from build123d import *

# Parameters (mm, degrees)
SKETCH1_W            = 103
SKETCH1_H            = 62.04
BOSS_EXTRUDE1_DEPTH  = 2
SKETCH2_W            = 103
SKETCH2_H            = 2
BOSS_EXTRUDE2_DEPTH  = 3
SKETCH5_W            = 8
SKETCH5_H            = 2.5
BOSS_EXTRUDE4_DEPTH  = 10
BOSS_EXTRUDE5_DEPTH  = 10
SKETCH7_R            = 1
CUT_EXTRUDE1_DEPTH   = 3
FILLET2_R            = 2
SKETCH8_W            = 103
SKETCH8_H            = 2.5
BOSS_EXTRUDE6_DEPTH  = 3
SKETCH9_W            = 8
SKETCH9_H            = 2.5
BOSS_EXTRUDE7_DEPTH  = 2
SKETCH11_R           = 1
CUT_EXTRUDE3_DEPTH   = 22
FILLET4_R            = 1
SKETCH12_W           = 12
SKETCH12_H           = 2.5
BOSS_EXTRUDE8_DEPTH  = 2
FILLET5_R            = 1
SKETCH13_R           = 0.95132711
CUT_EXTRUDE4_DEPTH   = 12
FILLET6_R            = 1
SKETCH14_W           = 103
SKETCH14_H           = 2.5
BOSS_EXTRUDE9_DEPTH  = 3
SKETCH15_W           = 8
SKETCH15_H           = 2.5
BOSS_EXTRUDE10_DEPTH = 5
SKETCH16_R           = 1
CUT_EXTRUDE5_DEPTH   = 15
FILLET7_R            = 1
CUT_EXTRUDE6_DEPTH   = 5


with BuildPart() as part:
    # Sketch1 → Boss-Extrude1 (new body)
    with BuildSketch(Plane(origin=(0, 0, 0), x_dir=(1, 0, 0), z_dir=(0, 1, 0))):
        Rectangle(SKETCH1_W, SKETCH1_H)
    extrude(amount=BOSS_EXTRUDE1_DEPTH)

    # Sketch2 → Boss-Extrude2 (add)
    with BuildSketch(Plane(origin=(0, 0, -31.02), x_dir=(-1, 0, 0), z_dir=(0, 0, -1))):
        with Locations((0, 1)):
            Rectangle(SKETCH2_W, SKETCH2_H)
    extrude(amount=BOSS_EXTRUDE2_DEPTH)

    # Sketch5 → Boss-Extrude4 (add)
    with BuildSketch(Plane(origin=(0, 2, 0), x_dir=(1, 0, 0), z_dir=(0, 1, 0))):
        with Locations((47.5, 29.77)):
            Rectangle(SKETCH5_W, SKETCH5_H)
    boss_extrude4 = extrude(amount=BOSS_EXTRUDE4_DEPTH)

    # Sketch6 → Boss-Extrude5 (add)
    with BuildSketch(Plane(origin=(0, 2, 0), x_dir=(1, 0, 0), z_dir=(0, 1, 0))):
        Polygon((43.5, 28.52), (0, 28.52), (0, 30.925842428), (43.5, 31.02), align=None)
    boss_extrude5 = extrude(amount=BOSS_EXTRUDE5_DEPTH)

    # Sketch7 → Cut-Extrude1 (cut)
    with BuildSketch(Plane.XY.offset(-28.52)):
        with Locations((47.5, 6)):
            Circle(SKETCH7_R)
    cut_extrude1 = extrude(amount=-CUT_EXTRUDE1_DEPTH, mode=Mode.SUBTRACT)

    # Mirror1: Boss-Extrude4, Boss-Extrude5, Cut-Extrude1 across plane
    add(boss_extrude4.mirror(Plane(origin=(0, 0, 0), x_dir=(0, 0, 1), z_dir=(1, 0, 0))))
    add(boss_extrude5.mirror(Plane(origin=(0, 0, 0), x_dir=(0, 0, 1), z_dir=(1, 0, 0))))
    add(cut_extrude1.mirror(Plane(origin=(0, 0, 0), x_dir=(0, 0, 1), z_dir=(1, 0, 0))), mode=Mode.SUBTRACT)

    # Fillet2
    fillet2_edges = [part.edges().sort_by_distance(p)[0] for p in [
        (0, 2, -28.52),
    ]]
    fillet(fillet2_edges, radius=FILLET2_R)

    # Sketch8 → Boss-Extrude6 (add)
    with BuildSketch(Plane(origin=(0, 2, 0), x_dir=(1, 0, 0), z_dir=(0, 1, 0))):
        with Locations((0, -3.73)):
            Rectangle(SKETCH8_W, SKETCH8_H)
    extrude(amount=BOSS_EXTRUDE6_DEPTH)

    # Sketch9 → Boss-Extrude7 (add)
    with BuildSketch(Plane(origin=(0, 5, 0), x_dir=(1, 0, 0), z_dir=(0, 1, 0))):
        with Locations((47.5, -3.73)):
            Rectangle(SKETCH9_W, SKETCH9_H)
    extrude(amount=BOSS_EXTRUDE7_DEPTH)

    # Sketch11 → Cut-Extrude3 (cut)
    with BuildSketch(Plane.XY.offset(4.98)):
        with Locations((47.13, 4.5)):
            Circle(SKETCH11_R)
    extrude(amount=-CUT_EXTRUDE3_DEPTH, mode=Mode.SUBTRACT)

    # Fillet4
    fillet4_edges = [part.edges().sort_by_distance(p)[0] for p in [
        (0, 2, 4.98),
    ]]
    fillet(fillet4_edges, radius=FILLET4_R)

    # Sketch12 → Boss-Extrude8 (add)
    with BuildSketch(Plane(origin=(0, 5, 0), x_dir=(1, 0, 0), z_dir=(0, 1, 0))):
        with Locations((-45.5, -3.73)):
            Rectangle(SKETCH12_W, SKETCH12_H)
    extrude(amount=BOSS_EXTRUDE8_DEPTH)

    # Fillet5
    fillet5_edges = [part.edges().sort_by_distance(p)[0] for p in [
        (-39.5, 5, 3.73),
    ]]
    fillet(fillet5_edges, radius=FILLET5_R)

    # Sketch13 → Cut-Extrude4 (cut)
    with BuildSketch(Plane.XY.offset(4.98)):
        with Locations((-44.5, 4.5)):
            Circle(SKETCH13_R)
    extrude(amount=-CUT_EXTRUDE4_DEPTH, mode=Mode.SUBTRACT)

    # Fillet6
    fillet6_edges = [part.edges().sort_by_distance(p)[0] for p in [
        (43.5, 5, 3.73),
    ]]
    fillet(fillet6_edges, radius=FILLET6_R)

    # Sketch14 → Boss-Extrude9 (add)
    with BuildSketch(Plane(origin=(0, 2, 0), x_dir=(1, 0, 0), z_dir=(0, 1, 0))):
        with Locations((0, -27.27)):
            Rectangle(SKETCH14_W, SKETCH14_H)
    extrude(amount=BOSS_EXTRUDE9_DEPTH)

    # Sketch15 → Boss-Extrude10 (add)
    with BuildSketch(Plane(origin=(0, 5, 0), x_dir=(1, 0, 0), z_dir=(0, 1, 0))):
        with Locations((47.5, -27.27)):
            Rectangle(SKETCH15_W, SKETCH15_H)
        with Locations((-47.5, -27.27)):
            Rectangle(SKETCH15_W, SKETCH15_H)
    extrude(amount=BOSS_EXTRUDE10_DEPTH)

    # Sketch16 → Cut-Extrude5 (cut)
    with BuildSketch(Plane.XY.offset(31.02)):
        with Locations((47.5, 6)):
            Circle(SKETCH16_R)
        with Locations((-47.5, 6)):
            Circle(SKETCH16_R)
    extrude(amount=-CUT_EXTRUDE5_DEPTH, mode=Mode.SUBTRACT)

    # Fillet7
    fillet7_edges = [part.edges().sort_by_distance(p)[0] for p in [
        (0, 2, 26.02),
        (43.5, 5, 27.27),
        (-43.5, 5, 27.27),
    ]]
    fillet(fillet7_edges, radius=FILLET7_R)

    # Sketch17 → Cut-Extrude6 (cut)
    with BuildSketch(Plane(origin=(0, 2, 0), x_dir=(1, 0, 0), z_dir=(0, 1, 0))):
        with BuildLine():
            Line((43.5, -22.121075172), (31.88534696, -22.121075172))
            ThreePointArc((31.88534696, -22.121075172), (30.471133397, -21.535288735), (29.88534696, -20.121075172))
            Line((29.88534696, -20.121075172), (29.88534696, -10.50434013))
            ThreePointArc((29.88534696, -10.50434013), (30.471133397, -9.090126568), (31.88534696, -8.50434013))
            Line((31.88534696, -8.50434013), (43.5, -8.50434013))
            ThreePointArc((43.5, -8.50434013), (44.914213562, -9.090126568), (45.5, -10.50434013))
            Line((45.5, -10.50434013), (45.5, -20.121075172))
            ThreePointArc((45.5, -20.121075172), (44.914213562, -21.535288735), (43.5, -22.121075172))
        make_face()
        with BuildLine():
            Line((25.88534696, -20.121075172), (25.88534696, -10.50434013))
            ThreePointArc((25.88534696, -10.50434013), (25.299560522, -9.090126568), (23.88534696, -8.50434013))
            Line((23.88534696, -8.50434013), (6.608652469, -8.50434013))
            ThreePointArc((6.608652469, -8.50434013), (5.194438907, -9.090126568), (4.608652469, -10.50434013))
            Line((4.608652469, -10.50434013), (4.608652469, -20.121075172))
            ThreePointArc((4.608652469, -20.121075172), (5.194438907, -21.535288735), (6.608652469, -22.121075172))
            Line((6.608652469, -22.121075172), (23.88534696, -22.121075172))
            ThreePointArc((23.88534696, -22.121075172), (25.299560522, -21.535288735), (25.88534696, -20.121075172))
        make_face()
        with BuildLine():
            Line((44.914213562, 19.849036172), (40.619219164, 24.14403057))
            ThreePointArc((40.619219164, 24.14403057), (39.970372466, 24.577576073), (39.205005602, 24.729817008))
            Line((39.205005602, 24.729817008), (34.780809577, 24.729817008))
            ThreePointArc((34.780809577, 24.729817008), (33.366596015, 24.14403057), (32.780809577, 22.729817008))
            Line((32.780809577, 22.729817008), (32.780809577, 15.003047088))
            ThreePointArc((32.780809577, 15.003047088), (33.366596015, 13.588833526), (34.780809577, 13.003047088))
            Line((34.780809577, 13.003047088), (43.5, 13.003047088))
            ThreePointArc((43.5, 13.003047088), (44.914213562, 13.588833526), (45.5, 15.003047088))
            Line((45.5, 15.003047088), (45.5, 18.43482261))
            ThreePointArc((45.5, 18.43482261), (45.347759065, 19.200189474), (44.914213562, 19.849036172))
        make_face()
        with BuildLine():
            Line((43.5, 10.003047088), (34.780809577, 10.003047088))
            ThreePointArc((34.780809577, 10.003047088), (33.366596015, 9.417260651), (32.780809577, 8.003047088))
            Line((32.780809577, 8.003047088), (32.780809577, 2))
            ThreePointArc((32.780809577, 2), (33.366596015, 0.585786438), (34.780809577, 0))
            Line((34.780809577, 0), (43.5, 0))
            ThreePointArc((43.5, 0), (44.914213562, 0.585786438), (45.5, 2))
            Line((45.5, 2), (45.5, 8.003047088))
            ThreePointArc((45.5, 8.003047088), (44.914213562, 9.417260651), (43.5, 10.003047088))
        make_face()
        with BuildLine():
            Line((28.780809577, 2), (28.780809577, 11.452131966))
            ThreePointArc((28.780809577, 11.452131966), (28.19502314, 12.866345529), (26.780809577, 13.452131966))
            Line((26.780809577, 13.452131966), (6.608652469, 13.452131966))
            ThreePointArc((6.608652469, 13.452131966), (5.194438907, 12.866345529), (4.608652469, 11.452131966))
            Line((4.608652469, 11.452131966), (4.608652469, 2))
            ThreePointArc((4.608652469, 2), (5.194438907, 0.585786438), (6.608652469, 0))
            Line((6.608652469, 0), (26.780809577, 0))
            ThreePointArc((26.780809577, 0), (28.19502314, 0.585786438), (28.780809577, 2))
        make_face()
        with BuildLine():
            Line((28.780809577, 19.452131966), (28.780809577, 22.729817008))
            ThreePointArc((28.780809577, 22.729817008), (28.19502314, 24.14403057), (26.780809577, 24.729817008))
            Line((26.780809577, 24.729817008), (6.608652469, 24.729817008))
            ThreePointArc((6.608652469, 24.729817008), (5.194438907, 24.14403057), (4.608652469, 22.729817008))
            Line((4.608652469, 22.729817008), (4.608652469, 19.452131966))
            ThreePointArc((4.608652469, 19.452131966), (5.194438907, 18.037918404), (6.608652469, 17.452131966))
            Line((6.608652469, 17.452131966), (26.780809577, 17.452131966))
            ThreePointArc((26.780809577, 17.452131966), (28.19502314, 18.037918404), (28.780809577, 19.452131966))
        make_face()
    cut_extrude6 = extrude(amount=-CUT_EXTRUDE6_DEPTH, mode=Mode.SUBTRACT)

    # Mirror4: Cut-Extrude6 across plane
    add(cut_extrude6.mirror(Plane(origin=(0, 0, 0), x_dir=(0, 0, 1), z_dir=(1, 0, 0))), mode=Mode.SUBTRACT)


solid = part.part
Model file for the job. Use its own axes, mm. A direction names the side the tool comes from. Give positions to 0.01 mm unless a question says otherwise; leave off trailing zeros. Loops run counter-clockwise (first coordinate to the right, second up) from the corner with the lowest first, then second, coordinate; pieces in that order, holes last.
1) Tool access for faces 1 (the flat face through (-1, 4, 28.52)), 2 (the flat face through (29.885, 1, 15)), 3 (the cylindrical face through (-45.45, 4.54, 3.75)): list every direction of +Z, -Z, +X, -X, +Y, -Y with a clear straight run to the whole face (end or side of a thin tool).
2) Wall check: line 1 (Z direction, x = -6.5, y = 1.25); line 2 (Z direction, x = -7.5, y = 1.5); line 3 (Z direction, x = -42.5, y = 4). Give the ranges that are in metal, low to high.
3) Saw through at A-A (y = 8.25). Write the cut outline in (x, z), plus the area to 3 significant figures.
4) Saw through at B-B (x = 12). Count the separate pieces of the cut face and the enclosed holes in it, plus the area to 3 significant figures.
5) Saw through at C-C (z = 14). Write the cut outline in (x, y), plus the area to 3 significant figures.
6) Pull direction Z, two halves, no side cores. Call faces 4 (the flat face through (46.6, 6.9, -31.02)), 5 (the flat face through (-48, 10, 27)), 6 (the flat face through (39, 1, -10.003)): +Z half, -Z half, draft (parallel to the pull), parting line (faces both ways), or undercut.
7) Flat gauge pins, fed straight in: pin 1 Ø5 at (x, y) = (18, 8) entering from -Z; pin 2 Ø1.2 at (x, z) = (4.5, 26.5) entering from +Y; pin 3 Ø2 at (x, y) = (6.5, 6.5) entering from -Z. Where does each tip first touch, or does it go through?
8) Saw through at D-D (x = -2). Write the cut outline in (y, z), plus the area to 3 significant figures.
Answer block:
1. face 1: +Z, +X, -X, +Y
1. face 2: +Y, -Y
1. face 3: none
2. line 1: z = -34.02 to -24.73, -17.46 to -13.45, 0 to 8.51, 22.12 to 31.02
2. line 2: z = -34.02 to -24.73, -17.45 to -13.45, 0 to 8.5, 22.12 to 31.02
2. line 3: z = -31.02 to -28.52, 2.48 to 4.98, 26.02 to 28.52
3. outline: (-51.5, -31.02) - (-43.5, -31.02) - (0, -30.93) - (43.5, -31.02) - (51.5, -31.02) - (51.5, -28.52) - (-51.5, -28.52) - close; (-51.5, 26.02) - (-43.5, 26.02) - (-43.5, 28.52) - (-51.5, 28.52) - close; (43.5, 26.02) - (51.5, 26.02) - (51.5, 28.52) - (43.5, 28.52) - close
3. area: 293 mm2
4. separate pieces: 4
4. enclosed holes: 0
4. area: 102 mm2
5. outline: (-51.5, 0) - (-45.5, 0) - (-45.5, 2) - (-51.5, 2) - close; (-29.89, 0) - (-25.89, 0) - (-25.89, 2) - (-29.89, 2) - close; (-4.61, 0) - (4.61, 0) - (4.61, 2) - (-4.61, 2) - close; (25.89, 0) - (29.89, 0) - (29.89, 2) - (25.89, 2) - close; (45.5, 0) - (51.5, 0) - (51.5, 2) - (45.5, 2) - close
5. area: 58.4 mm2
6. face 4: -Z half
6. face 5: draft
6. face 6: undercut
7. pin 1: stops at z = -30.97
7. pin 2: stops at y = 5
7. pin 3: stops at z = -30.94
8. outline: (0, -34.02) - (2, -34.02) - (2, -30.93) - (12, -30.93) - (12, -28.52) - (4, -28.52) arc R2 cw to (2, -26.52) - (2, 2.48) - (5, 2.48) - (5, 4.98) - (3, 4.98) arc R1 cw to (2, 5.98) - (2, 25.02) arc R1 cw to (3, 26.02) - (5, 26.02) - (5, 28.52) - (2, 28.52) - (2, 31.02) - (0, 31.02) - close
8. area: 170 mm2
